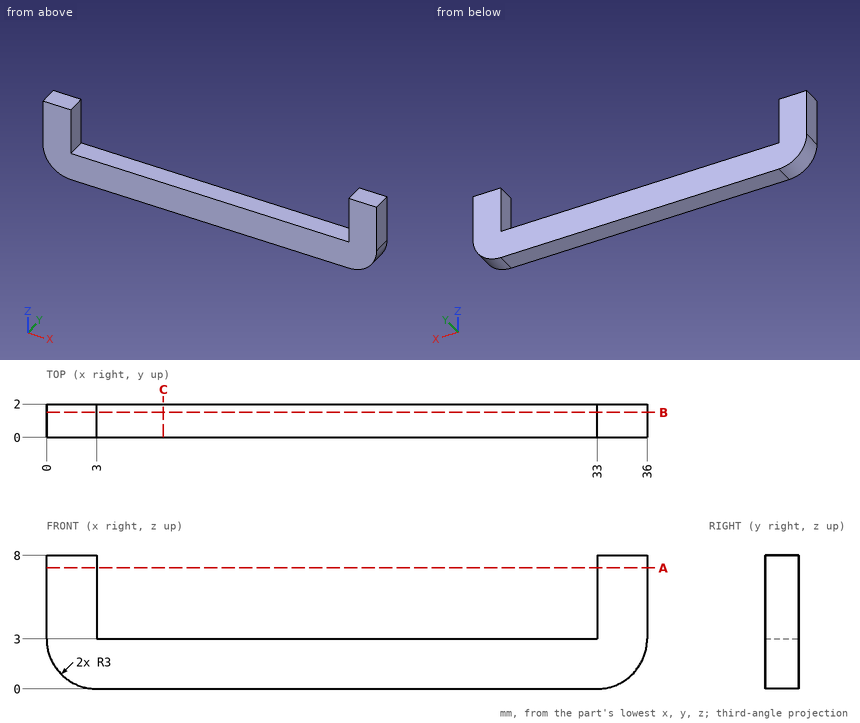
The drawing under review shows one solid part. Ordinate dimensions are in mm from its lowest x, y, z. Round coordinates to 2 decimals unless told otherwise and drop trailing zeros. Loops run counter-clockwise (first coordinate to the right, second up) from the corner with the lowest first, then second, coordinate; pieces in that order, holes last. Notation, with made-up numbers: (35.5, 35) - (78.5, 35) arc R27 ccw to (78.5, 69) - close; hole circle Ø1 at (-23, -11.5). An arc over 180 degrees is marked (long way). Use a Markdown table: item, result. Add a question column.
Q1. Add section A-A (z = 7.25). State the section outline as (x, y) points.
Q2. Add section B-B (y = 1.5). State the section outline as (x, z) points.
Q3. Add section C-C (x = 7). State the section outline as (y, z) points, plus the area to 3 significant figures.
Q4. For probe 1 along X at (y, z) = (0.6, 4); probe 2 along Z at (x, y) = (14.5, 0.55); probe 3 along Z at (x, y) = (34.5, 0.4), list the stretches that pass through material, from the lowest coordinate up.
Worked answers:
| question | item | result |
|---|---|---|
| 1 | outline | (0, 0) - (3, 0) - (3, 2) - (0, 2) - close; (33, 0) - (36, 0) - (36, 2) - (33, 2) - close |
| 2 | outline | (0, 3) arc R3 ccw to (3, 0) - (33, 0) arc R3 ccw to (36, 3) - (36, 8) - (33, 8) - (33, 3) - (3, 3) - (3, 8) - (0, 8) - close |
| 3 | outline | (0, 0) - (2, 0) - (2, 3) - (0, 3) - close |
| 3 | area | 6.00 mm² |
| 4 | probe 1 | 0 to 3, 33 to 36 |
| 4 | probe 2 | 0 to 3 |
| 4 | probe 3 | 0.4 to 8 |
